Source: CAD feature listing. Evaluate the final solid. Frame: model axes, mm. Round coordinates to 2 decimals unless told otherwise and drop trailing zeros. Write each loop counter-clockwise with the first axis right and the second up, starting at its lowest first coordinate (ties: lowest second). Pieces come first, ordered by that corner, then holes. Notation, with made-up numbers: M -27,-28 L -17,-28 A29 cw -17,-4 Z; hole C 31,10 d1. An arc over 180 degrees is marked long. Answer in a Markdown table with one row per item. Add a question column.
Item 1: Material intervals for probe 1 along Z at (x, y) = (66.75, 0.65); probe 2 along X at (y, z) = (0.55, 47.75); probe 3 along Y at (x, z) = (13.5, -14.5), sorted ascending.
Item 2: Contact query for flat-ended pins moving along their axis: pin 1 (0.5 mm diameter, centred on y = 2, z = 24, fed in from +X); pin 2 (5 mm diameter, centred on y = -4, z = -1, fed in from -X); pin 3 (3 mm diameter, centred on y = -4, z = 4.5, fed in from +X); pin 4 (3 mm diameter, centred on y = -2.5, z = 33, fed in from +X). Output: stop coordinate, or through.
Item 3: Cut plane C-C on z = -4. Return loops of the section in (x, y).
Item 4: Cut plane A-A on z = 47.75. Return loops of the section in (x, y), and give its area (3 significant figures).
Item 5: Cut plane B-B on x = 66.75. Return loops of the section in (y, z).
Item 6: Cut plane D-D on y = -1.75. Return loops of the section in (x, z), and give its area (3 significant figures).
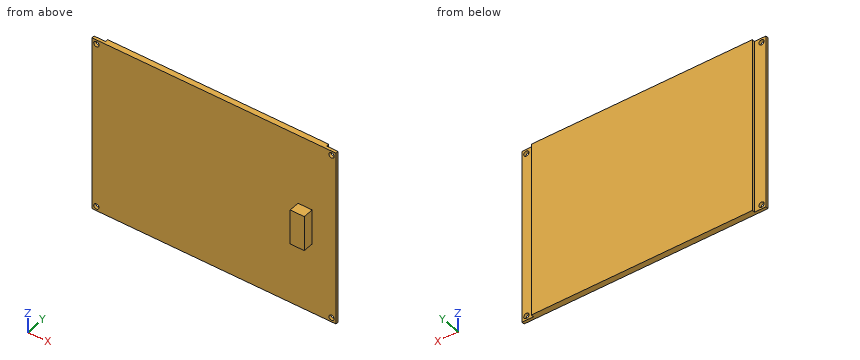
from build123d import *

# Parameters (mm, degrees)
SKETCH1_W           = 138.5
SKETCH1_H           = 100.5
SKETCH1_R           = 1.5
BOSS_EXTRUDE1_DEPTH = 1.6
SKETCH2_W           = 125.5
SKETCH2_H           = 100.5
BOSS_EXTRUDE2_DEPTH = 1.6
SKETCH3_W           = 8
SKETCH3_H           = 20
BOSS_EXTRUDE3_DEPTH = 6


with BuildPart() as part:
    # Sketch1 → Boss-Extrude1 (new body)
    with BuildSketch(Plane(origin=(0, 0, 0), x_dir=(1, 0, 0), z_dir=(0, 1, 0))):
        Rectangle(SKETCH1_W, SKETCH1_H)
        with Locations(Location((-66.75, 47.75, 0), (0, 0, 270))):
            Circle(SKETCH1_R, mode=Mode.SUBTRACT)
        with Locations(Location((66.75, 47.75, 0), (0, 0, 270))):
            Circle(SKETCH1_R, mode=Mode.SUBTRACT)
        with Locations(Location((66.75, -47.75, 0), (0, 0, 270))):
            Circle(SKETCH1_R, mode=Mode.SUBTRACT)
        with Locations(Location((-66.75, -47.75, 0), (0, 0, 270))):
            Circle(SKETCH1_R, mode=Mode.SUBTRACT)
    extrude(amount=BOSS_EXTRUDE1_DEPTH)

    # Sketch2 → Boss-Extrude2 (add)
    with BuildSketch(Plane(origin=(0, 1.6, 0), x_dir=(1, 0, 0), z_dir=(0, 1, 0))):
        Rectangle(SKETCH2_W, SKETCH2_H)
    extrude(amount=BOSS_EXTRUDE2_DEPTH)

    # Sketch3 → Boss-Extrude3 (add)
    with BuildSketch(Plane.XZ):
        with Locations((51.75, 0.25)):
            Rectangle(SKETCH3_W, SKETCH3_H)
    extrude(amount=BOSS_EXTRUDE3_DEPTH)


solid = part.part
Results below:
| question | item | result |
|---|---|---|
| 1 | probe 1 | -50.25 to -49.25, -46.25 to 46.25, 49.25 to 50.25 |
| 1 | probe 2 | -69.25 to -68.25, -65.25 to 65.25, 68.25 to 69.25 |
| 1 | probe 3 | 0 to 3.2 |
| 2 | pin 1 | x = 62.75 |
| 2 | pin 2 | x = 47.75 |
| 2 | pin 3 | x = 55.75 |
| 2 | pin 4 | through |
| 3 | outline | M -69.25,0 L 47.75,0 L 47.75,-6 L 55.75,-6 L 55.75,0 L 69.25,0 L 69.25,1.6 L 62.75,1.6 L 62.75,3.2 L -62.75,3.2 L -62.75,1.6 L -69.25,1.6 Z |
| 4 | outline | M -69.25,0 L -68.25,0 L -68.25,1.6 L -69.25,1.6 Z; M -65.25,0 L 65.25,0 L 65.25,1.6 L 62.75,1.6 L 62.75,3.2 L -62.75,3.2 L -62.75,1.6 L -65.25,1.6 Z; M 68.25,0 L 69.25,0 L 69.25,1.6 L 68.25,1.6 Z |
| 4 | area | 413 mm2 |
| 5 | outline | M 0,-50.25 L 1.6,-50.25 L 1.6,-49.25 L 0,-49.25 Z; M 0,-46.25 L 1.6,-46.25 L 1.6,46.25 L 0,46.25 Z; M 0,49.25 L 1.6,49.25 L 1.6,50.25 L 0,50.25 Z |
| 6 | outline | M 47.75,-9.75 L 55.75,-9.75 L 55.75,10.25 L 47.75,10.25 Z |
| 6 | area | 160 mm2 |
